Design review of the part built by this model. Coordinates are the model's own, in mm. Round coordinates to 2 decimals unless told otherwise and drop trailing zeros. Return JSON: item names as keys, results as strings. Group by question number.
from build123d import *

# Parameters (mm, degrees)
F0_W     = 235
F0_H     = 50
F0_R     = 2.1
F1_DEPTH = 3
F2_R     = 10
F3_R     = 2.5
F4_DEPTH = 3.001


with BuildPart() as f1:
    # F0 (on Top) → F1 (new body)
    with BuildSketch(Plane.XY):
        Rectangle(F0_W, F0_H)
        with Locations((-106.5, 0)):
            Circle(F0_R, mode=Mode.SUBTRACT)
        with Locations((106.5, 0)):
            Circle(F0_R, mode=Mode.SUBTRACT)
    extrude(amount=-F1_DEPTH)

    # F2
    f2_edges = [f1.edges().sort_by_distance(p)[0] for p in [
        (117.5, 25, -1.5),
        (117.5, -25, -1.5),
        (-117.5, -25, -1.5),
        (-117.5, 25, -1.5),
    ]]
    fillet(f2_edges, radius=F2_R)

    # F3 (on face) → F4 (cut, through all)
    with BuildSketch(Plane.XY):
        with Locations((-71.357113, 15.577964)):
            Circle(F3_R)
        with Locations((-26.3474, 15.577964)):
            Circle(F3_R)
        with Locations((71.357113, 15.577964)):
            Circle(F3_R)
        with Locations((26.3474, 15.577964)):
            Circle(F3_R)
        with Locations((71.357113, -15.577964)):
            Circle(F3_R)
        with Locations((-26.3474, -15.577964)):
            Circle(F3_R)
        with Locations((-71.357113, -15.577964)):
            Circle(F3_R)
        with Locations((26.3474, -15.577964)):
            Circle(F3_R)
    extrude(amount=-F4_DEPTH, mode=Mode.SUBTRACT)


solid = f1.part
Q1. Insertion check: pin 1 Ø1 at (y, z) = (16.5, -2) entering from +X. The pin has a flat end and moves straight along its axis. Give the tip position at first contact, or say it passes through.
Q2. For line 1 (Y direction, x = -26.5, z = -2.5); line 2 (X direction, y = -16, z = -0.4); line 3 (X direction, y = -15, z = -1.9), list the stretches that pass through material, from the lowest coordinate up.
Q3. Add section A-A, the plane z = -0.6. Give the number of separate pieces and of enclosed holes in the cut face, plus the area to 3 significant figures.
Evaluation:
{
 "1": {"pin 1": "x = 117.45"},
 "2": {"line 1": "-25 to -18.07, -13.08 to 13.08, 18.07 to 25", "line 2": "-117.45 to -73.82, -68.89 to -28.81, -23.88 to 23.88, 28.81 to 68.89, 73.82 to 117.45", "line 3": "-117.5 to -73.79, -68.92 to -28.78, -23.92 to 23.92, 28.78 to 68.92, 73.79 to 117.5"},
 "3": {"separate pieces": "1", "enclosed holes": "10", "area": "11,500 mm²"}
}
